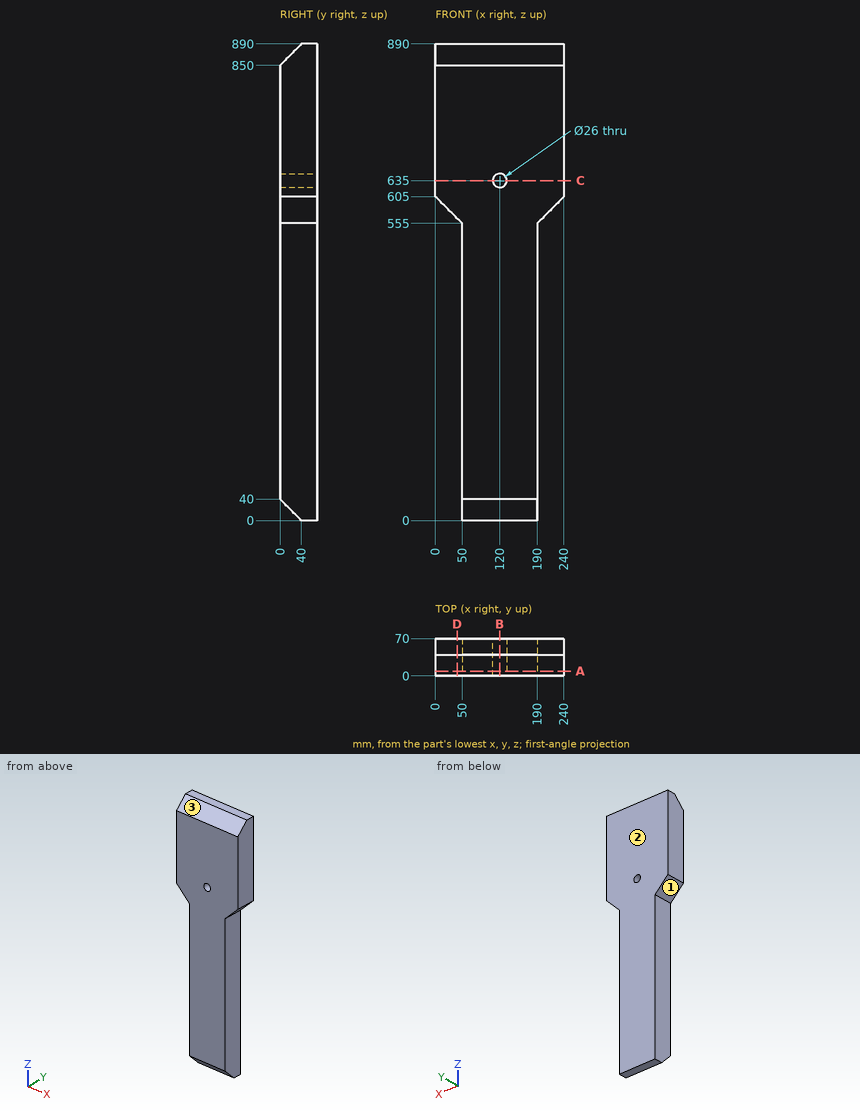
Check sheet for the drawn part. Datum: minimum x, y, z corner. Units: mm. Coordinates: 2 decimals unless noted, no trailing zeros. Loops run counter-clockwise (first coordinate to the right, second up) from the corner with the lowest first, then second, coordinate; pieces in that order, holes last. Notation, with made-up numbers: (87.25, -37.75) -> (141.25, -37.75) arc R12 ccw to (141.25, -17.75) -> close; hole circle Ø9 at (37, 42.5). An arc over 180 degrees is marked (long way). Answer as a JSON object with one key per item and string values. Group by question number.
Item 1: Depth check by flat-ended pin: pin 1 (8 mm diameter, centred on y = 16, z = 537, fed in from +X); pin 2 (4 mm diameter, centred on x = 35.5, y = 40, fed in from -Z); pin 3 (3 mm diameter, centred on x = 78, y = 17.5, fed in from +Z). Enter the tip coordinate at first touch or a pass-through.
Item 2: Sectioned sample at D-D on x = 40.5. Record the boundary of the cut face in (y, z), plus the area to 3 significant figures.
Item 3: Mould release check, pull along Z, two halves, no side actions. Record for the marked faces 1, 2 and 3: +Z half, -Z half, draft (parallel to the pull), parting line (faces both ways), or undercut.
Item 4: Sectioned sample at B-B on x = 120. Record the boundary of the cut face in (y, z).
Item 5: Scan lines: probe 1 along Z at (x, y) = (120, 50); probe 2 along X at (y, z) = (17.5, 635); probe 3 along X at (y, z) = (27, 504.5). Record each from-to range of solid material in increasing order.
Item 6: Sectioned sample at C-C on z = 635. Record the boundary of the cut face in (x, y), plus the area to 3 significant figures.
Item 7: Sectioned sample at A-A on y = 9. Record the boundary of the cut face in (x, z), plus the area to 3 significant figures.
Evaluation:
{
 "1": {"pin 1": "stops at x = 190", "pin 2": "stops at z = 567.5", "pin 3": "stops at z = 869"},
 "2": {"outline": "(0, 564.5) -> (70, 564.5) -> (70, 890) -> (40, 890) -> (0, 850) -> close", "area": "22,000 mm²"},
 "3": {"face 1": "-Z half", "face 2": "draft", "face 3": "+Z half"},
 "4": {"outline": "(0, 40) -> (40, 0) -> (70, 0) -> (70, 622) -> (0, 622) -> close; (0, 648) -> (70, 648) -> (70, 890) -> (40, 890) -> (0, 850) -> close"},
 "5": {"probe 1": "z = 0 to 622, 648 to 890", "probe 2": "x = 0 to 107, 133 to 240", "probe 3": "x = 50 to 190"},
 "6": {"outline": "(0, 0) -> (107, 0) -> (107, 70) -> (0, 70) -> close; (133, 0) -> (240, 0) -> (240, 70) -> (133, 70) -> close", "area": "15,000 mm²"},
 "7": {"outline": "(0, 605) -> (50, 555) -> (50, 31) -> (190, 31) -> (190, 555) -> (240, 605) -> (240, 859) -> (0, 859) -> close; hole circle Ø26 at (120, 635)", "area": "143,000 mm²"}
}
